Autodesk Inventor part; units mm, degrees
ref_plane "YZ Plane" through (0, 0, 0) normal (1, 0, 0) x (0, 1, 0)
ref_plane "XZ Plane" through (0, 0, 0) normal (0, 1, 0) x (-1, 0, 0)
ref_plane "XY Plane" through (0, 0, 0) normal (0, 0, 1) x (1, 0, 0)
sketch "スケッチ1" plane through (0, 0, 0) normal (0, 0, 1) x (1, 0, 0)
  circle A0 centre (0, 0) radius 80
  circle A1 centre (0, 0) radius 70
  dimension "d0" = 160
  dimension "d1" = 10
extrude "押し出し1" add sketch "スケッチ1" along normal blind 2
sketch "スケッチ2" plane through (0, 0, 2) normal (0, 0, 1) x (1, 0, 0)
  point P0 (0, 0)
  point P1 (0, 75)
  dimension "d4" = 75
hole "穴1" at (0, 75, 2) direction (0, 0, -1) diameter 3.5 end through all
pattern_circular "円形状パターン1" count 6 over 360 about axis through (0, 0, 0) along (0, 0, 1) of "穴1"
sketch "スケッチ3" plane through (0, 0, 2) normal (0, 0, 1) x (1, 0, 0)
  circle A0 centre (0, 0) radius 77
  circle A1 centre (0, 0) radius 73
  dimension "d15" = 154
  dimension "d16" = 146
extrude "押し出し2" add sketch "スケッチ3" along normal blind 2
sketch "スケッチ4" plane through (0, 0, 2) normal (0, 0, 1) x (1, 0, 0)
  circle A0 centre (0, 0) radius 70
  circle A1 centre (0, 0) radius 80
  line L0 (5, -69.8212) -> (-5, -69.8212)
  line L1 (-5, -69.8212) -> (-5, -79.8436)
  line L2 (-5, -79.8436) -> (5, -79.8436)
  line L3 (5, -79.8436) -> (5, -69.8212)
  dimension "d19" = 10
extrude "押し出し3" cut sketch "スケッチ4" along normal blind 2 contours A0 L3 L2 L1
pattern_circular "円形状パターン2" count 6 over 360 about axis through (0, 0, 0) along (0, 0, 1) of "押し出し3"
properties part number "外周ピン抑え"
Check sheet for the modelled part. Datum: model origin and axes. Units: mm. A direction names the side the tool comes from. Coordinates: 2 decimals unless noted, no trailing zeros. Order: outer loops, then holes, each group sorted by start corner. A loop starts at its lowest first (then second) coordinate and runs counter-clockwise, first axis right, second up. Notation, with made-up numbers: (39, 59.25) -> (69, 59.25) arc R18 cw to (69, 87.25) -> close; hole circle Ø4 at (77.25, 69). An arc over 180 degrees is marked (long way). Write item = value, one per line. Start each with the question number.
1) Access from +Z, -Z, +X, -X, +Y, -Y to the whole of each face (thin tool, end or side, straight path). Record for faces 1 (the cylindrical face through (77, 0, 3)), 2 (the cylindrical face through (-36.1, -63.45, 2.99)), 3 (the cylindrical face through (38.07, 66.93, 2.99)), 4 (the cylindrical face through (-55.55, 42.594, 0.986)), 5 (the flat face through (-74, 0, 4)).
2) Go/stop test with flat-tipped pins: P1, Ø3, axis at x = -64.95, y = 37.5, coming from the -Z side; P2, Ø4.5, axis at x = 64.95, y = -37.5, coming from the -Z side. Record where each tip stops, or that it passes through.
3) Cross-section at B-B (x = 39). Enter the section's corners in (y, z), then the cut area to 3 significant figures.
4) Cross-section at A-A (y = 0). Enter the section's corners in (x, z), then the cut area to 3 significant figures.
5) Cross-section at C-C (z = 1.3). Enter the section's corners in (x, y) (3 decimals).
6) Mould release check, pull along Y, two halves, no side actions. Record for faces 6 (the cylindrical face through (-64.282, -39.117, 0.986)), 7 (the cylindrical face through (-38.927, 66.435, 2.986)), 8 (the flat face through (37, 64, 4)): +Y half, -Y half, draft (parallel to the pull), parting line (faces both ways), or undercut.
7) Material ranges on L1, parallel to X at y = -37.5, z = 0.6; L2, parallel to Y at x = -52.5, z = 0.8; L3, parallel to Y at x = -30, z = 2.7, recorded low to high.
Ans:
q1.face_1 = +Z, +X
q1.face_2 = +Z
q1.face_3 = +Z, +X, +Y
q1.face_4 = +Z, -Z
q1.face_5 = +Z, +X, -X, +Y, -Y
q2.P1 = through
q2.P2 = 0
q3.outline = (-69.85, 0) -> (-58.13, 0) -> (-58.13, 2) -> (-61.71, 2) -> (-61.71, 4) -> (-66.39, 4) -> (-66.39, 2) -> (-69.85, 2) -> close; (58.13, 0) -> (69.85, 0) -> (69.85, 2) -> (66.39, 2) -> (66.39, 4) -> (61.71, 4) -> (61.71, 2) -> (58.13, 2) -> close
q3.area = 65.6 mm²
q4.outline = (-80, 0) -> (-70, 0) -> (-70, 2) -> (-73, 2) -> (-73, 4) -> (-77, 4) -> (-77, 2) -> (-80, 2) -> close; (70, 0) -> (80, 0) -> (80, 2) -> (77, 2) -> (77, 4) -> (73, 4) -> (73, 2) -> (70, 2) -> close
q4.area = 56.0 mm²
q5.outline = circle Ø160 at (0, 0); hole circle Ø140 at (0, 0); hole circle Ø3.5 at (-64.952, -37.5); hole circle Ø3.5 at (-64.952, 37.5); hole circle Ø3.5 at (0, -75); hole circle Ø3.5 at (0, 75); hole circle Ø3.5 at (64.952, -37.5); hole circle Ø3.5 at (64.952, 37.5)
q6.face_6 = undercut
q6.face_7 = +Y half
q6.face_8 = draft
q7.L1 = -70.67 to -66.7, -63.2 to -59.11, 59.11 to 63.2, 66.7 to 70.67
q7.L2 = -60.36 to -46.3, 46.3 to 60.36
q7.L3 = -70.92 to -66.55, 66.55 to 70.92
